Design review of the part built by this model. Coordinates are the model's own, in mm. A direction names the side the tool comes from. Coordinates: 2 decimals unless noted, no trailing zeros. Write each loop counter-clockwise with the first axis right and the second up, starting at its lowest first coordinate (ties: lowest second). Pieces come first, ordered by that corner, then holes.
Q1. Clearance check with flat-ended pins moving along their axes: pin 1 Ø4 at (x, y) = (0, 0) entering from +Z; pin 2 Ø1.5 at (y, z) = (-2, 9) entering from -X; pin 3 Ø1.5 at (x, z) = (-1.5, 5.5) entering from -Y; pin 4 Ø5 at (x, z) = (-7.5, 4.5) entering from -Y. State where each tip first meets the part, or that it passes through.
Q2. Add section A-A, the plane y = 0. Give the boundary of the cut face in (x, z).
Q3. To check wall thickness, follow probe 1 along Y at (x, z) = (0, 3.75); probe 2 along Z at (x, y) = (-9.75, 5); probe 3 along X at (y, z) = (-1.5, 4). State the ranges of each line that lie inside material, in increasing order.
Q4. Machinability: for faces 5 (the face through (2, -9, 10.5)), 6 (the face through (-2.38, -10.74, 11.24)), which of the approach directions +Z, -Z, +X, -X, +Y, -Y give a long, thin tool a straight path to every point of the face, cutting with its end or side? Answer none if there is none.
Q5. The part is to be moulded in two halves that separate along Z. For faces 1 (the face through (-3, 0, 12)), 2 (the face through (-0.54, -2.44, 6.08)), 3 (the face through (-1.172, 8.923, 5.937)), 4 (the face through (2, -9, 1.5)), say which applies: +Z half, -Z half, draft (parallel to the pull), parting line (faces both ways), or undercut.
Q6. Add section C-C, the plane z = 8.5. Give the boundary of the cut face in (x, y), plus the area to 3 significant figures.
Q7. Add section D-D, the plane x = -5. Give the boundary of the cut face in (y, z).
from build123d import *

# Parameters (mm, degrees)
ESQUISSE1_R                  = 11
BOSS_EXTRU_1_DEPTH           = 1.5
ESQUISSE2_R                  = 9
BOSS_EXTRU_2_DEPTH           = 9
ESQUISSE3_R                  = 11
BOSS_EXTRU_3_DEPTH           = 1.5
ESQUISSE4_R                  = 2.5
ENL_V_MAT_EXTRU_1_DEPTH      = 1
ENL_V_MAT_EXTRU_1_DEPTH_BACK = 13


with BuildPart() as part:
    # Esquisse1 → Boss.-Extru.1 (new body)
    with BuildSketch(Plane.XY):
        Circle(ESQUISSE1_R)
    extrude(amount=BOSS_EXTRU_1_DEPTH)

    # Esquisse2 → Boss.-Extru.2 (add)
    with BuildSketch(Plane.XY.offset(1.5)):
        Circle(ESQUISSE2_R)
    extrude(amount=BOSS_EXTRU_2_DEPTH)

    # Esquisse3 → Boss.-Extru.3 (add)
    with BuildSketch(Plane.XY.offset(10.5)):
        Circle(ESQUISSE3_R)
    extrude(amount=BOSS_EXTRU_3_DEPTH)

    # Esquisse4 → Enlèv. mat.-Extru.1 (cut, two sides)
    with BuildSketch(Plane.XY.offset(12)) as enl_v_mat_extru_1_sk:
        Circle(ESQUISSE4_R)
    extrude(amount=ENL_V_MAT_EXTRU_1_DEPTH, mode=Mode.SUBTRACT)
    extrude(enl_v_mat_extru_1_sk.sketch, amount=-ENL_V_MAT_EXTRU_1_DEPTH_BACK, mode=Mode.SUBTRACT)


solid = part.part
Here are the results:
1. pin 1: passes through
1. pin 2: stops at x = -8.91
1. pin 3: stops at y = -8.97
1. pin 4: stops at y = -7.48
2. outline: (-11, 0) - (-2.5, 0) - (-2.5, 12) - (-11, 12) - (-11, 10.5) - (-9, 10.5) - (-9, 1.5) - (-11, 1.5) - close; (2.5, 0) - (11, 0) - (11, 1.5) - (9, 1.5) - (9, 10.5) - (11, 10.5) - (11, 12) - (2.5, 12) - close
3. probe 1: y = -9 to -2.5, 2.5 to 9
3. probe 2: z = 0 to 1.5, 10.5 to 12
3. probe 3: x = -8.87 to -2, 2 to 8.87
4. face 5: none
4. face 6: +Z, -Z
5. face 1: +Z half
5. face 2: draft
5. face 3: undercut
5. face 4: undercut
6. outline: circle Ø18 at (0, 0); hole circle Ø5 at (0, 0)
6. area: 235 mm2
7. outline: (-9.8, 0) - (9.8, 0) - (9.8, 1.5) - (7.48, 1.5) - (7.48, 10.5) - (9.8, 10.5) - (9.8, 12) - (-9.8, 12) - (-9.8, 10.5) - (-7.48, 10.5) - (-7.48, 1.5) - (-9.8, 1.5) - close
